from build123d import *

# Parameters (mm, degrees)
SKETCH_2_W          = 5
SKETCH_2_H          = 32
EXTRUDE_1_DEPTH     = 10
CUT_EXTRUDE_1_DEPTH = 34.619190948
SKETCH_4_R          = 0.8
CUT_EXTRUDE_2_DEPTH = 25.328165537


with BuildPart() as part:
    # 草图2 → 凸台-拉伸1 (new body)
    with BuildSketch(Plane(origin=(0, 0, 0), x_dir=(1, 0, 0), z_dir=(0, 1, 0))):
        with Locations((0, -16)):
            Rectangle(SKETCH_2_W, SKETCH_2_H)
    extrude(amount=EXTRUDE_1_DEPTH)

    # 草图3 → 切除-拉伸1 (cut, through all)
    with BuildSketch(Plane(origin=(0, 10, 0), x_dir=(1, 0, 0), z_dir=(0, 1, 0))):
        Polygon((2.5, -18.660254038), (1.25, -13.995190528), (-1.1, -21.85857128), (-2.5, -15), (-2.5, -32), (2.5, -32), align=None)
        Polygon((2.5, 0), (-2.5, 0), (1.25, -13.995190528), (2.5, -18.660254038), align=None)
    extrude(amount=-CUT_EXTRUDE_1_DEPTH, mode=Mode.SUBTRACT)

    # 草图4 → 切除-拉伸2 (cut, through all)
    with BuildSketch(Plane.ZY.offset(2.5)):
        with Locations((5, 5)):
            Circle(SKETCH_4_R)
        with Locations((10, 5)):
            Circle(SKETCH_4_R)
    extrude(amount=-CUT_EXTRUDE_2_DEPTH, mode=Mode.SUBTRACT)


solid = part.part
Here's how the part is built. I have some questions about the finished solid (model axes, mm). Give positions to 0.01 mm unless a question says otherwise; leave off trailing zeros. Write each loop counter-clockwise with the first axis right and the second up, starting at its lowest first coordinate (ties: lowest second). Pieces come first, ordered by that corner, then holes. Notation, with made-up numbers: (-5.5, 47.25) -> (21.5, 47.25) arc R22 ccw to (21.5, 81.25) -> close; hole circle Ø3 at (71, -5.75). An arc over 180 degrees is marked (long way). Use one line per item in the form item = value. Start each with the question number.
1. Imagine slicing it at C-C on x = -1.4. List the corners of the cut face in (y, z) for me.
2. Imagine slicing it at D-D on x = -0.3. List the corners of the cut face in (y, z) for me.
3. If I drill on L1, parallel to Y at x = -0.5, z = 10; L2, parallel to X at y = 1.5, z = 14; L3, parallel to X at y = 6, z = 1.5, over which ranges is the centre line in solid material (lowest first)?
4. Thinking about a two-plate mould opening in Z: for faces 1 (the face through (0.09, 5.07, 17.87)), 2 (the face through (-1.073, 4.694, 10.739)), 3 (the face through (-2.5, 5, 8)), which applies, +Z half, -Z half, draft (parallel to the pull), parting line (faces both ways), or undercut?
5. Imagine slicing it at A-A on z = 5. List the corners of the cut face in (x, y) for me, plus the area to 3 significant figures.
6. Will this pin go through, and if not, where does the flat tip stop? pin 1 Ø2 at (x, z) = (0, 6.5) entering from -Y.
7. Imagine slicing it at B-B on y = 5. List the corners of the cut face in (x, z) for me, plus the area to 3 significant figures.
Entries:
q1.outline = (0, 4.11) -> (10, 4.11) -> (10, 20.39) -> (0, 20.39) -> close; hole circle Ø1.6 at (5, 5); hole circle Ø1.6 at (5, 10)
q2.outline = (0, 8.21) -> (10, 8.21) -> (10, 19.18) -> (0, 19.18) -> close; hole circle Ø1.6 at (5, 10)
q3.L1 = 0 to 4.2, 5.8 to 10
q3.L2 = -2.5 to 1.25
q3.L3 = -2.5 to -2.1
q4.face_1 = +Z half
q4.face_2 = undercut
q4.face_3 = draft
q5.outline = (-2.5, 0) -> (-1.16, 0) -> (-1.16, 4.2) -> (-2.5, 4.2) -> close; (-2.5, 5.8) -> (-1.16, 5.8) -> (-1.16, 10) -> (-2.5, 10) -> close
q5.area = 11.3 mm²
q6.pin_1 = 0
q7.outline = (-2.5, 0) -> (-1.37, 4.2) -> (-2.5, 4.2) -> close; (-2.5, 5.8) -> (-0.95, 5.8) -> (-0.03, 9.2) -> (-2.5, 9.2) -> close; (-2.5, 10.8) -> (0.39, 10.8) -> (1.25, 14) -> (-1.1, 21.86) -> (-2.5, 15) -> close
q7.area = 35.3 mm²
